Work out the finished part from the listing and answer in its coordinate system (mm). A direction names the side the tool comes from. Round coordinates to 2 decimals unless told otherwise and drop trailing zeros. Order: outer loops, then holes, each group sorted by start corner. A loop starts at its lowest first (then second) coordinate and runs counter-clockwise, first axis right, second up. Notation, with made-up numbers: (-27, 70.25) - (24, 70.25) arc R17 ccw to (24, 87.25) - close; hole circle Ø11 at (51.5, 62.25). An arc over 180 degrees is marked (long way). Use one line per item in the form item = value. Start each with the question number.
Q1. The part is cut by section B-B on x = 13. Determine the outline of the cut face in (y, z).
Q2. Find the intervals of material crossed by line 1 (Z direction, x = 24, y = 122); line 2 (Z direction, x = 12.5, y = 114.5); line 3 (Y direction, x = -1, z = 24.5), in increasing order. Write a range as [from, to].
Q3. Given P1, Ø8, axis at x = 10.5, z = 41, coming from the +Y side; P2, Ø5, axis at x = 12, y = 114, coming from the +Z side; P3, Ø4, axis at y = 96, z = 30.5, coming from the +X side; P4, Ø12, axis at x = 15.5, z = 34.5, coming from the -Y side, each flat-ended and moving along its own axis, determine where each tip first touches the part or whether it passes through.
Q4. Which of the six approach directions +Z, -Z, +X, -X, +Y, -Y give full straight-line access (tool end or side, diameter ignored) to faces 1 (the flat face through (13.585, 95.808, 24.118)), 2 (the flat face through (27.678, 122, 24)), 3 (the flat face through (22, 127.678, 24)), 4 (the flat face through (24.192, 113.585, 24.118)), 5 (the flat face through (-4.093, 113.486, 24.118))?
Q5. For a pull along Z with two mould halves and no side action, classify faces 6 (the flat face through (13.486, 124.093, 24.118)), 7 (the cylindrical face through (6, 113, 31)), 8 (the flat face through (10, 110, 21.653)) as +Z half, -Z half, draft (parallel to the pull), parting line (faces both ways), or undercut.
Q6. The part is cut by section C-C on y = 118.5. Determine the outline of the cut face in (x, z).
Q7. The part is cut by section D-D on z = 27.5. Determine the outline of the cut face in (x, y), plus the area to 3 significant figures.
Q8. The part is cut by section A-A on y = 104. Determine the outline of the cut face in (x, z).
from build123d import *

# Parameters (mm, degrees)
CYLINDER011_R            = 5
CYLINDER011_DEPTH        = 15
PAD_DEPTH                = 5
ARRAY006_COUNT           = 4
CLONE017_PLACEMENT_ANGLE = 45


with BuildPart() as cylinder011:
    # Cylinder011 → Cylinder011 (new body)
    with BuildSketch(Plane.XY):
        Circle(CYLINDER011_R)
    extrude(amount=CYLINDER011_DEPTH)


with BuildPart() as sphere:
    # Sphere → Sphere (revolve)
    with BuildSketch(Plane(origin=(0, 0, 17), x_dir=(1, 0, 0), z_dir=(0, -1, 0))):
        with BuildLine():
            ThreePointArc((0, -6.5), (6.5, 0), (0, 6.5))
            Line((0, 6.5), (0, -6.5))
        make_face()
    revolve(axis=Axis((0, 0, 17), (0, 0, 1)))


with BuildPart() as obj1:
    # Sketch → Pad (new body)
    with BuildSketch(Plane.XY):
        Polygon((0, 7.5), (17.5, 7.5), (25, 0), (17.5, -7.5), (0, -7.5), align=None)
    extrude(amount=PAD_DEPTH)

    # Array006: obj1 ×4 about axis
    array006_axis = Axis((0, 0, 0), (0, 0, 1))


with BuildPart() as obj1_1:
    add(obj1.part)
    for i in range(1, ARRAY006_COUNT):
        add(obj1.part.rotate(array006_axis, i * 360 / ARRAY006_COUNT))

    # Fusion017: union Cylinder011, Sphere
    add(cylinder011.part)
    add(sphere.part)


with BuildPart() as obj1_2:
    # Clone017 placement: moved
    add(obj1_1.part.moved(Location((10, 110, 21.6533))).rotate(Axis((10, 110, 21.6533), (0, 0, 1)), CLONE017_PLACEMENT_ANGLE))


solid = obj1_2.part
Found:
q1.outline = (96.39, 21.65) - (123.61, 21.65) - (123.61, 26.65) - (114, 26.65) - (114, 34.5) arc R5.77 ccw (long way) to (106, 34.5) - (106, 26.65) - (96.39, 26.65) - close
q2.line_1 = [21.65, 26.65]
q2.line_2 = [21.65, 26.65], [34.68, 42.62]
q2.line_3 = [92.32, 109.61], [110.39, 127.68]
q3.P1 = 116.5
q3.P2 = 44.85
q3.P3 = through
q3.P4 = 103.56
q4.face_1 = +Z, -Z, -Y
q4.face_2 = +Z, -Z, +X, +Y, -Y
q4.face_3 = +Z, -Z, +X, -X, +Y
q4.face_4 = +Z, -Z, +X
q4.face_5 = +Z, -Z, -X
q5.face_6 = draft
q5.face_7 = undercut
q5.face_8 = -Z half
q6.outline = (-7.68, 21.65) - (27.68, 21.65) - (27.68, 26.65) - (-7.68, 26.65) - close
q7.outline = circle Ø10 at (10, 110)
q7.area = 78.5 mm²
q8.outline = (-6.61, 21.65) - (26.61, 21.65) - (26.61, 26.65) - (-6.61, 26.65) - close; circle Ø5 at (10, 38.65)
